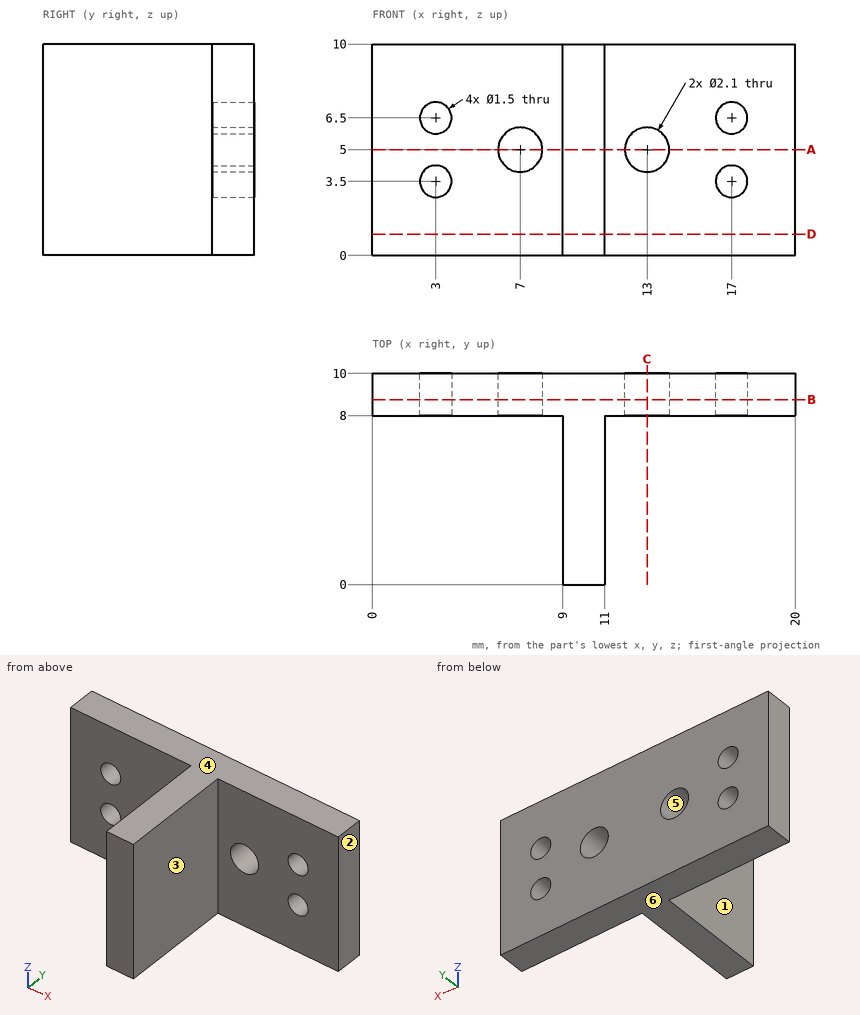
Study the drawing (mm; zero at the part's minimum x, y, z) and answer. A direction names the side the tool comes from. Give positions to 0.01 mm unless a question says otherwise; leave off trailing zeros. Order: outer loops, then holes, each group sorted by start corner. A loop starts at its lowest first (then second) coordinate and runs counter-clockwise, first axis right, second up.
1) For the marked faces 1, 2 and 3, determine the directions among +Z, -Z, +X, -X, +Y, -Y from which every point of the face is accessible in a straight line to the end or side of a thin tool.
Reported:
face 1: +Z, -Z, -X, -Y
face 2: +Z, -Z, +X, +Y, -Y
face 3: +Z, -Z, +X, -Y
2) Given P1, Ø1, axis at x = 5, z = 4.5, coming from the -Y side; P2, Ø1.2, axis at x = 17, z = 6.5, coming from the +Y side; P3, Ø4, axis at y = 5.5, z = 1, coming from the -X side, each flat-ended and moving along its own axis, determine where each tip first touches the part or whether it passes through.
Reported:
P1: stops at y = 8
P2: passes through
P3: stops at x = 9
3) Consider line 1 along Z through (x, y) = (3, 8.5); line 2 along Z through (x, y) = (7, 8.4); line 3 along X through (y, z) = (9, 7). Determine where each line is inside the solid, lowest interval first.
Reported:
line 1: z = 0 to 2.75, 4.25 to 5.75, 7.25 to 10
line 2: z = 0 to 3.95, 6.05 to 10
line 3: x = 0 to 2.44, 3.56 to 16.44, 17.56 to 20
4) Find section A-A on z = 5. Write down the section's boundary in (x, y), then the cut area to 3 significant figures.
Reported:
outline: (0, 8) - (5.95, 8) - (5.95, 10) - (0, 10) - close; (8.05, 8) - (9, 8) - (9, 0) - (11, 0) - (11, 8) - (11.95, 8) - (11.95, 10) - (8.05, 10) - close; (14.05, 8) - (20, 8) - (20, 10) - (14.05, 10) - close
area: 47.6 mm2
5) Find section B-B on y = 8.75. Write down the section's boundary in (x, z).
Reported:
outline: (0, 0) - (20, 0) - (20, 10) - (0, 10) - close; hole circle Ø1.5 at (3, 3.5); hole circle Ø1.5 at (3, 6.5); hole circle Ø2.1 at (7, 5); hole circle Ø2.1 at (13, 5); hole circle Ø1.5 at (17, 3.5); hole circle Ø1.5 at (17, 6.5)
6) Find section C-C on x = 13. Write down the section's boundary in (y, z), then the cut area to 3 significant figures.
Reported:
outline: (8, 0) - (10, 0) - (10, 3.95) - (8, 3.95) - close; (8, 6.05) - (10, 6.05) - (10, 10) - (8, 10) - close
area: 15.8 mm2
7) Determine the mould class of the marked faces 4, 5 and 6 for opening direction Z: pulls with the +Z half, pulls with the -Z half, needs draft (parallel to the pull), parting line crosses it, or undercut.
Reported:
face 4: pulls with the +Z half
face 5: undercut
face 6: pulls with the -Z half
8) Find section D-D on z = 1. Write down the section's boundary in (x, y).
Reported:
outline: (0, 8) - (9, 8) - (9, 0) - (11, 0) - (11, 8) - (20, 8) - (20, 10) - (0, 10) - close
